Check sheet for the modelled part. Datum: model origin and axes. Units: mm. A direction names the side the tool comes from. Give positions to 0.01 mm unless a question says otherwise; leave off trailing zeros. Write each loop counter-clockwise with the first axis right and the second up, starting at its lowest first coordinate (ties: lowest second). Pieces come first, ordered by that corner, then holes. Notation, with made-up numbers: (69, 66) -> (117, 66) arc R13 ccw to (117, 71) -> close; hole circle Ø7 at (3.25, 79.5). An arc over 180 degrees is marked (long way). Return JSON: item names as keys, results as strings.
from build123d import *

# Parameters (mm, degrees)
SKETCH_R        = 4
PAD_DEPTH       = 15
SKETCH001_R     = 3
POCKET_DEPTH    = 12
SKETCH002_R     = 1.8
POCKET001_DEPTH = 1.8
SKETCH003_W     = 30
SKETCH003_H     = 15
POCKET002_DEPTH = 13
POCKET004_DEPTH = 19


with BuildPart() as part:
    # Sketch → Pad (new body)
    with BuildSketch(Plane.XY):
        with BuildLine():
            ThreePointArc((-7.83079, 13.621483), (-10, 9.5), (-7.83079, 5.378516))
            Line((0, 0), (-7.83079, 5.378516))
            Line((34, 0), (0, 0))
            Line((41.830773, 5.378541), (34, 0))
            ThreePointArc((41.830773, 5.378541), (43.999947, 9.5), (41.830774, 13.621459))
            Line((34, 19), (41.830774, 13.621459))
            Line((0, 19), (34, 19))
            Line((-7.83079, 13.621483), (0, 19))
        make_face()
        with Locations((9.5, 9.5)):
            Circle(SKETCH_R, mode=Mode.SUBTRACT)
        with Locations((24.5, 9.5)):
            Circle(SKETCH_R, mode=Mode.SUBTRACT)
    extrude(amount=PAD_DEPTH)

    # Sketch001 → Pocket (cut)
    with BuildSketch(Plane(origin=(0, 0, 0), x_dir=(1, 0, 0), z_dir=(0, 0, -1))):
        with Locations((-5, -9.5)):
            Circle(SKETCH001_R)
        with Locations((39, -9.5)):
            Circle(SKETCH001_R)
    extrude(amount=-POCKET_DEPTH, mode=Mode.SUBTRACT)

    # Sketch002 → Pocket001 (cut)
    with BuildSketch(Plane.XY.offset(15)):
        with Locations((-5, 9.5)):
            Circle(SKETCH002_R)
        with Locations((39, 9.5)):
            Circle(SKETCH002_R)
    extrude(amount=-POCKET001_DEPTH, mode=Mode.SUBTRACT)

    # Sketch003 → Pocket002 (cut)
    with BuildSketch(Plane.XY.offset(15)):
        with Locations((17, 9.5)):
            Rectangle(SKETCH003_W, SKETCH003_H)
    extrude(amount=-POCKET002_DEPTH, mode=Mode.SUBTRACT)

    # Sketch004 → Pocket004 (cut)
    with BuildSketch(Plane.XZ):
        Polygon((-11, 13), (-11, -2), (45, -2), (45, 13), (44, 13), (34, 0), (0, 0), (-10, 13), align=None)
    extrude(amount=-POCKET004_DEPTH, mode=Mode.SUBTRACT)


solid = part.part
(1) Depth check by flat-ended pin: pin 1 Ø3 at (x, y) = (-5, 9.5) entering from -Z; pin 2 Ø6 at (y, z) = (8, 7.5) entering from -X; pin 3 Ø1.8 at (x, y) = (-5.5, 10) entering from +Z. Enter the tip coordinate at first touch or a pass-through.
Reply:
{"pin 1": "z = 12", "pin 2": "x = -8.08", "pin 3": "z = 13.2"}
(2) Release check for a two-part mould opening along X. For faces 4 (the flat face through (-2.71, 7.26, 3.52)), 5 (the flat face through (17, 19, 7)), 6 (the flat face through (17, 10, 2)) record: pulls with the +X half, pulls with the -X half, needs draft (parallel to the pull), parting line crosses it, or undercut.
Reply:
{"face 4": "pulls with the -X half", "face 5": "needs draft", "face 6": "undercut"}
(3) Cross-section at A-A on x = 9.5. Enter the section's corners in (y, z).
Reply:
{"outline": "(0, 0) -> (5.5, 0) -> (5.5, 2) -> (2, 2) -> (2, 15) -> (0, 15) -> close; (13.5, 0) -> (19, 0) -> (19, 15) -> (17, 15) -> (17, 2) -> (13.5, 2) -> close"}
(4) Set-up check for faces 1 (the flat face through (17, 0, 7)), 2 (the flat face through (32, 9, 9)), 3 (the cylindrical face through (-2.14, 8.6, 8.28)): record each of +Z, -Z, +X, -X, +Y, -Y from which the full face is reachable in a straight line by a thin tool's end or side.
Reply:
{"face 1": "+Z, -Z, +X, -X, -Y", "face 2": "+Z", "face 3": "-Z"}
(5) Cross-section at D-D on x = 29.5. Enter the section's corners in (y, z), then the cut area to 3 significant figures.
Reply:
{"outline": "(0, 0) -> (19, 0) -> (19, 15) -> (17, 15) -> (17, 2) -> (2, 2) -> (2, 15) -> (0, 15) -> close", "area": "90.0 mm^2"}
(6) Thickness scan on L1, parallel to X at y = 9.5, z = 9.5; L2, parallel to Y at x = 9.5, z = 0.5; L3, parallel to Y at x = 23.5, z = 3. Record the ranges inside material, lowest first.
Reply:
{"L1": "-2 to 2, 32 to 36", "L2": "0 to 5.5, 13.5 to 19", "L3": "0 to 2, 17 to 19"}
(7) Cross-section at C-C on z = 6.5. Enter the section's corners in (x, y).
Reply:
{"outline": "(-5, 3.43) -> (0, 0) -> (34, 0) -> (39, 3.43) -> (39, 6.5) arc R3 cw to (39, 12.5) -> (39, 15.57) -> (34, 19) -> (0, 19) -> (-5, 15.57) -> (-5, 12.5) arc R3 cw to (-5, 6.5) -> close; hole (2, 2) -> (32, 2) -> (32, 17) -> (2, 17) -> close"}
(8) Cross-section at B-B on y = 9.5. State how many separate pieces and enclosed holes the cut face has, then the cut area to 3 significant figures.
Reply:
{"separate pieces": "3", "enclosed holes": "0", "area": "179 mm^2"}
